from build123d import *

# Parameters (mm, degrees)
MODEL_W                 = 3
MODEL_H                 = 3
SALIENTE_EXTRUIR1_DEPTH = 3


with BuildPart() as part:
    # Model → Saliente-Extruir1 (new body)
    with BuildSketch(Plane.XY):
        with BuildLine():
            Line((16.117442786, 300.002712349), (52.117442786, 300.002712349))
            ThreePointArc((52.117442786, 300.002712349), (55.299423301, 298.684692865), (56.617442786, 295.502712349))
            Line((56.617442786, 295.502712349), (56.617442786, 259.502712349))
            ThreePointArc((56.617442786, 259.502712349), (55.299423301, 256.320731834), (52.117442786, 255.002712349))
            Line((52.117442786, 255.002712349), (16.117442786, 255.002712349))
            ThreePointArc((16.117442786, 255.002712349), (12.935462271, 256.320731834), (11.617442786, 259.502712349))
            Line((11.617442786, 259.502712349), (11.617442786, 295.502712349))
            ThreePointArc((11.617442786, 295.502712349), (12.935462271, 298.684692865), (16.117442786, 300.002712349))
        make_face()
        with Locations((16.117442786, 295.502712349)):
            Rectangle(MODEL_W, MODEL_H, mode=Mode.SUBTRACT)
        with Locations((25.117442786, 295.502712349)):
            Rectangle(MODEL_W, MODEL_H, mode=Mode.SUBTRACT)
        with Locations((34.117442786, 295.502712349)):
            Rectangle(MODEL_W, MODEL_H, mode=Mode.SUBTRACT)
        with Locations((43.117442786, 295.502712349)):
            Rectangle(MODEL_W, MODEL_H, mode=Mode.SUBTRACT)
        with Locations((52.117442786, 295.502712349)):
            Rectangle(MODEL_W, MODEL_H, mode=Mode.SUBTRACT)
        with Locations((16.117442786, 259.502712349)):
            Rectangle(MODEL_W, MODEL_H, mode=Mode.SUBTRACT)
        with Locations((25.117442786, 259.502712349)):
            Rectangle(MODEL_W, MODEL_H, mode=Mode.SUBTRACT)
        with Locations((34.117442786, 259.502712349)):
            Rectangle(MODEL_W, MODEL_H, mode=Mode.SUBTRACT)
        with Locations((43.117442786, 259.502712349)):
            Rectangle(MODEL_W, MODEL_H, mode=Mode.SUBTRACT)
        with Locations((52.117442786, 259.502712349)):
            Rectangle(MODEL_W, MODEL_H, mode=Mode.SUBTRACT)
        with Locations((16.117442786, 286.502712349)):
            Rectangle(MODEL_W, MODEL_H, mode=Mode.SUBTRACT)
        with Locations((25.117442786, 286.502712349)):
            Rectangle(MODEL_W, MODEL_H, mode=Mode.SUBTRACT)
        with Locations((34.117442786, 286.502712349)):
            Rectangle(MODEL_W, MODEL_H, mode=Mode.SUBTRACT)
        with Locations((43.117442786, 286.502712349)):
            Rectangle(MODEL_W, MODEL_H, mode=Mode.SUBTRACT)
        with Locations((52.117442786, 286.502712349)):
            Rectangle(MODEL_W, MODEL_H, mode=Mode.SUBTRACT)
        with Locations((16.117442786, 277.502712349)):
            Rectangle(MODEL_W, MODEL_H, mode=Mode.SUBTRACT)
        with Locations((25.117442786, 277.502712349)):
            Rectangle(MODEL_W, MODEL_H, mode=Mode.SUBTRACT)
        with Locations((34.117442786, 277.502712349)):
            Rectangle(MODEL_W, MODEL_H, mode=Mode.SUBTRACT)
        with Locations((43.117442786, 277.502712349)):
            Rectangle(MODEL_W, MODEL_H, mode=Mode.SUBTRACT)
        with Locations((52.117442786, 277.502712349)):
            Rectangle(MODEL_W, MODEL_H, mode=Mode.SUBTRACT)
        with Locations((16.117442786, 268.502712349)):
            Rectangle(MODEL_W, MODEL_H, mode=Mode.SUBTRACT)
        with Locations((25.117442786, 268.502712349)):
            Rectangle(MODEL_W, MODEL_H, mode=Mode.SUBTRACT)
        with Locations((34.117442786, 268.502712349)):
            Rectangle(MODEL_W, MODEL_H, mode=Mode.SUBTRACT)
        with Locations((43.117442786, 268.502712349)):
            Rectangle(MODEL_W, MODEL_H, mode=Mode.SUBTRACT)
        with Locations((52.117442786, 268.502712349)):
            Rectangle(MODEL_W, MODEL_H, mode=Mode.SUBTRACT)
    extrude(amount=SALIENTE_EXTRUIR1_DEPTH)


solid = part.part
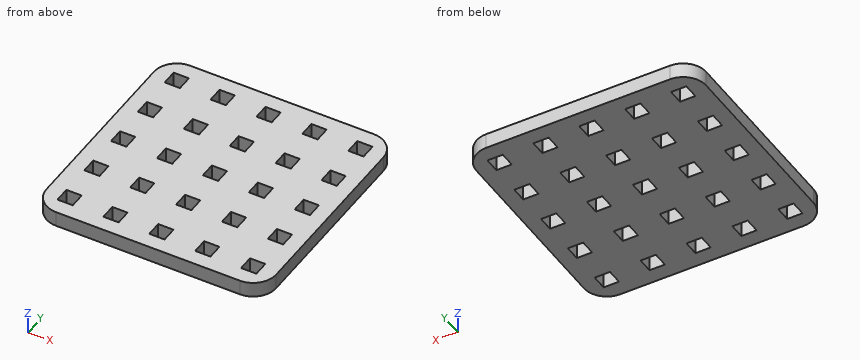
For this review, take the finished solid that the model builds, in its own axes (mm). Give positions to 0.01 mm unless a question says otherwise; leave off trailing zeros. Loops run counter-clockwise (first coordinate to the right, second up) from the corner with the lowest first, then second, coordinate; pieces in that order, holes last.
Item 1: Take a section at B-B, the plane z = 1.9. Give the number of separate pieces and of enclosed holes in the cut face, and give its area (3 significant figures).
Item 2: Take a section at A-A, the plane x = 34.5. State the section outline as (y, z) points.
Item 3: For line 1 along X through (y, z) = (295.5, 1.35); line 2 along Y through (x, z) = (24, 2.5); line 3 along Y through (x, z) = (15, 2), list the stretches that pass through material, from the lowest coordinate up.
Calculated:
1. separate pieces: 1
1. enclosed holes: 25
1. area: 1,780 mm2
2. outline: (255, 0) - (258, 0) - (258, 3) - (255, 3) - close; (261, 0) - (267, 0) - (267, 3) - (261, 3) - close; (270, 0) - (276, 0) - (276, 3) - (270, 3) - close; (279, 0) - (285, 0) - (285, 3) - (279, 3) - close; (288, 0) - (294, 0) - (294, 3) - (288, 3) - close; (297, 0) - (300, 0) - (300, 3) - (297, 3) - close
3. line 1: x = 11.62 to 14.62, 17.62 to 23.62, 26.62 to 32.62, 35.62 to 41.62, 44.62 to 50.62, 53.62 to 56.62
3. line 2: y = 255 to 258, 261 to 267, 270 to 276, 279 to 285, 288 to 294, 297 to 300
3. line 3: y = 255.14 to 258, 261 to 267, 270 to 276, 279 to 285, 288 to 294, 297 to 299.86
